Source: CAD feature listing. Evaluate the final solid. Frame: model axes, mm. Face numbers are marked on the shaded views. Give positions to 0.01 mm unless a question says otherwise; leave off trailing zeros. Answer in a Markdown table with one row per item. Add a question column.
(1) Material intervals for line 1 along X through (y, z) = (-104, 4.25); line 2 along X through (y, z) = (-139, 3.75); line 3 along Z through (x, y) = (27.5, -132), sorted ascending.
(2) Mould query, pull axis Z, two halves, no side actions, for the marked faces 1 and 2. Classes: pulls with the +Z half, pulls with the -Z half, needs draft (parallel to the pull), parting line crosses it, or undercut.
(3) Pin query (flat end, axial travel): P1, Ø1.2, axis at x = -8.5, y = -149, coming from the -Z side; P2, Ø10, axis at x = -24, y = -157, coming from the -Z side; P3, Ø9, axis at x = 3.5, y = -105, coming from the +Z side; P4, Ø1, axis at x = -14, z = -3, coming from the +Y side. Return the tip coordinate at first contact, or that it passes through.
from build123d import *

# Parameters (mm, degrees)
F1_DEPTH = 200


# Not quite as in the source:
# - ends of sketch curves that miss each other by under 0.0002 mm in the source are joined


with BuildPart() as f1:
    # F0 (on Front) → F1 (new body)
    with BuildSketch(Plane.XZ):
        with BuildLine():
            Line((-18.103784, -0.791851), (-17.32476, -2.14116))
            ThreePointArc((-17.32476, -2.14116), (-16.7014064944, -1.7527534112), (-16.1728328101, -1.2428131594))
            Line((-16.1728328101, -1.2428131594), (16.172833, -1.242813))
            ThreePointArc((16.172833, -1.242813), (16.7014064944, -1.7527534112), (17.3247602013, -2.1411595856))
            Line((17.3247602013, -2.1411595856), (18.103784, -0.791851))
            ThreePointArc((18.103784, -0.791851), (18.853784, 2.007187), (19.6037840458, -0.7918510793))
            Line((19.6037840458, -0.7918510793), (20.382808, -2.14116))
            ThreePointArc((20.382808, -2.14116), (21.820396824, -0.8500174455), (22.353784, 1.007187))
            Line((22.353784, 1.007187), (22.353784, 4.007187))
            Line((22.353784, 4.007187), (28.65, 4.007187))
            Line((28.65, 4.007187), (28.65, 0.916375))
            Line((28.65, 0.916375), (24.995488, -2.738136))
            ThreePointArc((24.995488, -2.738136), (24.7787154675, -3.8279264324), (25.702595, -4.445243))
            Line((25.702595, -4.445243), (27.714112, -4.445243))
            Line((27.714112, -4.445243), (25.365346, -8.705386))
            Line((25.365346, -8.705386), (26.54757, -9.357187))
            Line((26.54757, -9.357187), (29.182471, -4.578059))
            ThreePointArc((29.182471, -4.578059), (29.1678006221, -3.5867237514), (28.30675, -3.095243))
            Line((28.30675, -3.095243), (27.754677, -3.095243))
            ThreePointArc((27.754677, -3.095243), (27.292737369, -2.7865850428), (27.4011231094, -2.2416901094))
            Line((27.4011231094, -2.2416901094), (29.707107, 0.064294))
            ThreePointArc((29.707107, 0.064294), (29.9238795325, 0.3887175676), (30, 0.771401))
            Line((30, 0.771401), (30, 8.357187))
            ThreePointArc((30, 8.357187), (29.7071067812, 9.0642937812), (29, 9.357187))
            Line((29, 9.357187), (24.5, 9.357187))
            Line((24.5, 9.357187), (24.5, 8.007187))
            Line((24.5, 8.007187), (28.65, 8.007187))
            Line((28.65, 8.007187), (28.65, 5.357187))
            Line((28.65, 5.357187), (12.5, 5.357187))
            Line((12.5, 5.357187), (12.5, 4.107187))
            Line((12.5, 4.107187), (14, 4.107187))
            Line((14, 4.107187), (14.125, 0.107187))
            Line((14.125, 0.107187), (7.875, 0.107187))
            Line((7.875, 0.107187), (8, 4.107187))
            Line((8, 4.107187), (9.5, 4.107187))
            Line((9.5, 4.107187), (9.5, 5.357187))
            Line((9.5, 5.357187), (1.5, 5.357187))
            Line((1.5, 5.357187), (1.5, 4.107187))
            Line((1.5, 4.107187), (3, 4.107187))
            Line((3, 4.107187), (3.125, 0.107187))
            Line((3.125, 0.107187), (-3.125, 0.107187))
            Line((-3.125, 0.107187), (-3, 4.107187))
            Line((-3, 4.107187), (-1.5, 4.107187))
            Line((-1.5, 4.107187), (-1.5, 5.357187))
            Line((-1.5, 5.357187), (-9.5, 5.357187))
            Line((-9.5, 5.357187), (-9.5, 4.107187))
            Line((-9.5, 4.107187), (-8, 4.107187))
            Line((-8, 4.107187), (-7.875, 0.107187))
            Line((-7.875, 0.107187), (-14.125, 0.107187))
            Line((-14.125, 0.107187), (-14, 4.107187))
            Line((-14, 4.107187), (-12.5, 4.107187))
            Line((-12.5, 4.107187), (-12.5, 5.357187))
            Line((-12.5, 5.357187), (-28.65, 5.357187))
            Line((-28.65, 5.357187), (-28.65, 8.007187))
            Line((-28.65, 8.007187), (-24.5, 8.007187))
            Line((-24.5, 8.007187), (-24.5, 9.357187))
            Line((-24.5, 9.357187), (-29, 9.357187))
            ThreePointArc((-29, 9.357187), (-29.7071067812, 9.0642937812), (-30, 8.357187))
            Line((-30, 8.357187), (-30, 0.771401))
            ThreePointArc((-30, 0.771401), (-29.9238795325, 0.3887175676), (-29.7071067812, 0.0642942188))
            Line((-29.7071067812, 0.0642942188), (-27.401123, -2.24169))
            ThreePointArc((-27.401123, -2.24169), (-27.2927362337, -2.7865847162), (-27.754676, -3.095243))
            Line((-27.754676, -3.095243), (-28.306749, -3.095243))
            ThreePointArc((-28.306749, -3.095243), (-29.1677994994, -3.5867235436), (-29.1824708638, -4.5780589249))
            Line((-29.1824708638, -4.5780589249), (-26.54757, -9.357187))
            Line((-26.54757, -9.357187), (-25.365345, -8.705386))
            Line((-25.365345, -8.705386), (-27.714112, -4.445243))
            Line((-27.714112, -4.445243), (-25.702595, -4.445243))
            ThreePointArc((-25.702595, -4.445243), (-24.7787154675, -3.8279264324), (-24.9954882188, -2.7381362188))
            Line((-24.9954882188, -2.7381362188), (-28.65, 0.916375))
            Line((-28.65, 0.916375), (-28.65, 4.007187))
            Line((-28.65, 4.007187), (-22.353784, 4.007187))
            Line((-22.353784, 4.007187), (-22.353784, 1.007187))
            ThreePointArc((-22.353784, 1.007187), (-21.820396824, -0.8500174455), (-20.3828077987, -2.1411595856))
            Line((-20.3828077987, -2.1411595856), (-19.603784, -0.791851))
            ThreePointArc((-19.603784, -0.791851), (-18.853784, 2.007187), (-18.103784, -0.791851))
        make_face()
    extrude(amount=F1_DEPTH)


solid = f1.part
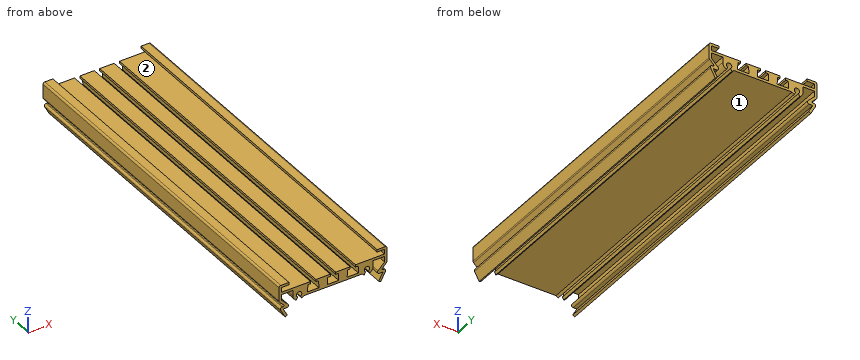
Values follow:
| question | item | result |
|---|---|---|
| 1 | line 1 | x = -30 to -12.5, -9.5 to -1.5, 1.5 to 9.5, 12.5 to 30 |
| 1 | line 2 | x = -30 to -28.65, -22.35 to -14.01, -7.99 to -3.01, 3.01 to 7.99, 14.01 to 22.35, 28.65 to 30 |
| 1 | line 3 | z = -7.63 to -4.83, -4.45 to -3.03, -2.14 to -0.23, 4.01 to 5.36, 8.01 to 9.36 |
| 2 | face 1 | pulls with the -Z half |
| 2 | face 2 | undercut |
| 3 | P1 | stops at z = -1.24 |
| 3 | P2 | stops at z = -9.36 |
| 3 | P3 | stops at z = 5.36 |
| 3 | P4 | passes through |
